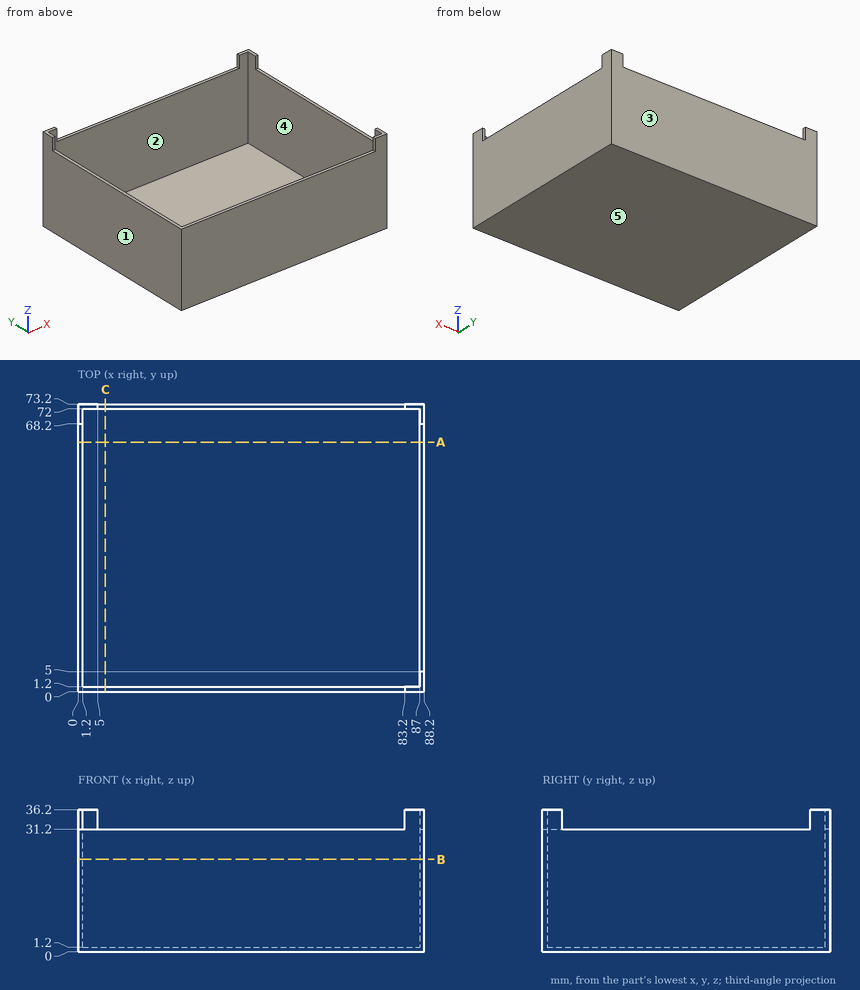
Design review of the part shown in the three views and the two pictorial views. Dimensions are in mm from the part's minimum x, y and z. A direction names the side the tool comes from. Coordinates: 2 decimals unless noted, no trailing zeros. Order: outer loops, then holes, each group sorted by start corner. A loop starts at its lowest first (then second) coordinate and runs counter-clockwise, first axis right, second up. Notation, with made-up numbers: (36.25, 46.25) - (82.25, 46.25) arc R36 cw to (82.25, 84.25) - close; hole circle Ø7 at (35.25, -19.5). An arc over 180 degrees is marked (long way). One line per question, with ' | ' between items.
Q1. Consider section A-A, the plane y = 63.5. Give the boundary of the cut face in (x, z).
Answer key:
outline: (0, 0) - (88.2, 0) - (88.2, 31.2) - (87, 31.2) - (87, 1.2) - (1.2, 1.2) - (1.2, 31.2) - (0, 31.2) - close
Q2. Consider section B-B, the plane z = 23.5. Give the boundary of the cut face in (x, y), then the cut area to 3 significant figures.
Answer key:
outline: (0, 0) - (88.2, 0) - (88.2, 73.2) - (0, 73.2) - close; hole (1.2, 1.2) - (87, 1.2) - (87, 72) - (1.2, 72) - close | area: 382 mm2
Q3. For the marked faces 1 and 2, list the 3-axis set-ups (+Z, -Z, +X, -X, +Y, -Y) from which the entire face can be reached by the end or side of a thin tool; tool diameter is ignored.
Answer key:
face 1: +Z, -Z, -X, +Y, -Y | face 2: +Z
Q4. The part is to be moulded in two halves that separate along Y. For the marked faces 3, 4 and 5, say which applies: +Y half, -Y half, draft (parallel to the pull), parting line (faces both ways), or undercut.
Answer key:
face 3: +Y half | face 4: undercut | face 5: draft
Q5. Clearance check with flat-ended pins moving along their axes: pin 1 Ø21 at (x, y) = (65.5, 22.5) entering from +Z; pin 2 Ø0.6 at (x, y) = (87.5, 41) entering from +Z; pin 3 Ø1.3 at (x, z) = (0.5, 35) entering from -Y. State where each tip first meets the part, or that it passes through.
Answer key:
pin 1: stops at z = 1.2 | pin 2: stops at z = 31.2 | pin 3: stops at y = 68.2
Q6. Consider section C-C, the plane x = 7. Give the boundary of the cut face in (y, z).
Answer key:
outline: (0, 0) - (73.2, 0) - (73.2, 31.2) - (72, 31.2) - (72, 1.2) - (1.2, 1.2) - (1.2, 31.2) - (0, 31.2) - close
Q7. To check wall thickness, follow line 1 along X through (y, z) = (19, 20); line 2 along Y through (x, z) = (37.5, 11); line 3 along Z through (x, y) = (10.5, 65). State the ranges of each line that lie inside material, in increasing order.
Answer key:
line 1: x = 0 to 1.2, 87 to 88.2 | line 2: y = 0 to 1.2, 72 to 73.2 | line 3: z = 0 to 1.2
